Geometry check sheet. Reference: the model listing, model coordinates, mm. Face numbers are marked on the shaded views. A direction names the side the tool comes from. Coordinates: 2 decimals unless noted, no trailing zeros. Loops run counter-clockwise (first coordinate to the right, second up) from the corner with the lowest first, then second, coordinate; pieces in that order, holes last. Notation, with made-up numbers: (-2.75, 78) - (12.25, 78) arc R36 cw to (12.25, 114) - close; hole circle Ø4 at (51.5, -9). An arc over 180 degrees is marked (long way). Write item = value, one per line. Start each with the question number.
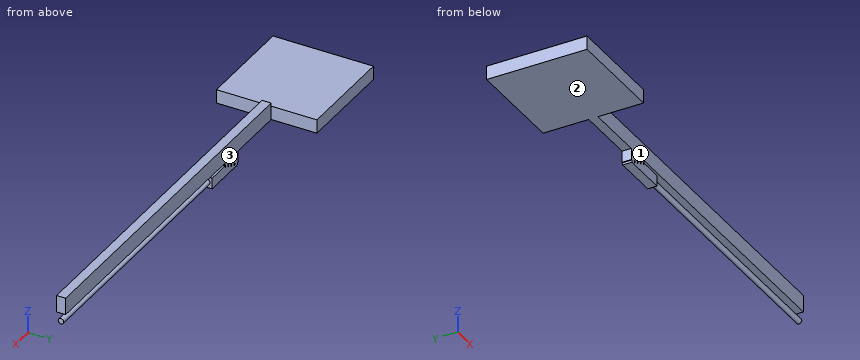
from build123d import *

# Parameters (mm, degrees)
F2_W      = 203.2
F2_H      = 5.08
F3_DEPTH  = 9.398
F0_W      = 12.7
F0_H      = 5.08
F12_DEPTH = 7.62
F11_W     = 0.508
F11_H     = 1.524
F11_H_2   = 1.27
F13_DEPTH = 2.54
F15_W     = 55.88
F15_H     = 55.88
F16_DEPTH = 7.62
F17_DEPTH = 6.096
F18_R     = 1.524


# Not quite as in the source:
# - a feature names something its author has since deleted; it is built from what else it names


with BuildPart() as f3:
    # F2 (on offset) → F3 (new body)
    with BuildSketch(Plane.XY.offset(7.62)):
        with Locations((43.18, 4.064)):
            Rectangle(F2_W, F2_H)
    extrude(amount=F3_DEPTH)

    # F0 (on Top) → F12 (join)
    with BuildSketch(Plane.XY):
        with Locations((-19.05, 4.064)):
            Rectangle(F0_W, F0_H)
    extrude(amount=F12_DEPTH)

    # F11 (on offset) → F13 (cut, symmetric)
    with BuildSketch(Plane.XZ.offset(-4.064)):
        with Locations((-12.954, 5.842)):
            Rectangle(F11_W, F11_H)
        with Locations((-25.146, 0.635)):
            Rectangle(F11_W, F11_H_2)
        with Locations((-19.05, 3.175)):
            Rectangle(F11_W, F11_H_2)
        with Locations((-16.002, 4.445)):
            Rectangle(F11_W, F11_H_2)
        with Locations((-22.098, 1.905)):
            Rectangle(F11_W, F11_H_2)
    extrude(amount=F13_DEPTH, both=True, mode=Mode.SUBTRACT)

    # F15 (on offset) → F16 (join)
    with BuildSketch(Plane.XY.offset(7.62)):
        with Locations((-86.36, 4.064)):
            Rectangle(F15_W, F15_H)
    extrude(amount=F16_DEPTH)

    # F0 (on Top) → F17 (join)
    with BuildSketch(Plane.XY):
        Polygon((-6.35, 1.524), (0, 1.524), (0, 6.604), (-12.7, 6.604), (-12.7, 1.524), align=None)
    extrude(amount=F17_DEPTH)

    # F21: sweep along a path in F20
    with BuildLine(Plane.XZ.offset(-3.9624)) as f21_path:
        Line((0, 3.048), (144.78, 3.048))
    # F18 (on Right) → F21 (sweep)
    with BuildSketch(Plane.YZ):
        with Locations((3.9624, 3.048)):
            Circle(F18_R)
    sweep(path=f21_path.line)


solid = f3.part
(1) Scan lines: line 1 (Z direction, x = -63, y = -15); line 2 (Y direction, x = 45.5, z = 12); line 3 (X direction, y = -2, z = 11). Record each from-to range of solid material in increasing order.
(2) Depth check by flat-ended pin: pin 1 (0.6 mm diameter, centred on y = 5, z = 1.5, fed in from +X); pin 2 (0.8 mm diameter, centred on y = 4, z = 5.5, fed in from -X); pin 3 (6 mm diameter, centred on y = 24, z = 11.5, fed in from +X). Enter the tip coordinate at first touch or a pass-through.
(3) Sectioned sample at A-A on z = 10.25. Enter the section's corners in (x, y).
(4) Sectioned sample at C-C on x = 63. Enter the section's corners in (y, z).
(5) Sectioned sample at D-D on x = -37. Enter the section's corners in (y, z), plus the area to 3 significant figures.
(6) Sectioned sample at B-B on y = -6.5. Enter the section's corners in (x, z).
(7) Tool access check on the marked faces 1, 2 and 3. Record the directions out of +Z, -Z, +X, -X, +Y, -Y that give a thin tool (end or side, any length) a straight path to the whole face; none if there is none.
Working result:
q1.line_1 = 7.62 to 15.24
q1.line_2 = 1.52 to 6.6
q1.line_3 = -114.3 to -58.42
q2.pin_1 = 0
q2.pin_2 = -25.4
q2.pin_3 = -58.42
q3.outline = (-114.3, -23.88) - (-58.42, -23.88) - (-58.42, 1.52) - (144.78, 1.52) - (144.78, 6.6) - (-58.42, 6.6) - (-58.42, 32) - (-114.3, 32) - close
q4.outline = (1.52, 7.62) - (6.6, 7.62) - (6.6, 17.02) - (1.52, 17.02) - close; circle Ø3.05 at (3.96, 3.05)
q5.outline = (1.52, 7.62) - (6.6, 7.62) - (6.6, 17.02) - (1.52, 17.02) - close
q5.area = 47.7 mm2
q6.outline = (-114.3, 7.62) - (-58.42, 7.62) - (-58.42, 15.24) - (-114.3, 15.24) - close
q7.face_1 = +Z, -Z, +X, -Y
q7.face_2 = -Z, -X, +Y, -Y
q7.face_3 = +Z, -Z, +X, +Y
